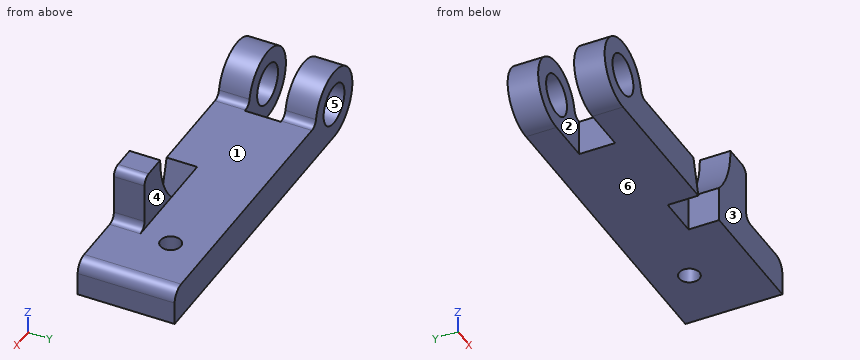
```python
from build123d import *

# Parameters (mm, degrees)
F0_R     = 0.5
F1_DEPTH = 1.1875
F2_W     = 2.274463
F2_H     = 0.879
F2_R     = 0.25
F3_DEPTH = 2.251
F5_DEPTH = 1.625
F7_DEPTH = 0.75
F8_R     = 0.2


with BuildPart() as f1:
    # F0 (on Front) → F1 (new body, symmetric)
    with BuildSketch(Plane.XZ):
        Polygon((-4.03, 0), (-3.03, 0), (-3.03, 0.88), (-4.266, 0.88), align=None)
        with BuildLine():
            Line((-7.646, 0), (-4.03, 0))
            Line((-4.03, 0), (-4.266, 0.88))
            Line((-4.266, 0.88), (-6.58468, 0.88))
            ThreePointArc((-6.58468, 0.88), (-6.712337, 0.92604), (-6.781221, 1.042963))
            ThreePointArc((-6.781221, 1.042963), (-8.323424, 1.441691), (-7.646, 0))
        make_face()
        with Locations((-7.646, 0.88)):
            Circle(F0_R, mode=Mode.SUBTRACT)
        with BuildLine():
            Line((-3.03, 0), (0, 0))
            Line((0, 0), (0, 0.57))
            ThreePointArc((0, 0.57), (-0.090797, 0.789203), (-0.31, 0.88))
            Line((-0.31, 0.88), (-1.737, 0.88))
            Line((-1.737, 0.88), (-1.737, 2.05))
            ThreePointArc((-1.737, 2.05), (-1.795579, 2.191421), (-1.937, 2.25))
            Line((-1.937, 2.25), (-2.487, 2.25))
            ThreePointArc((-2.487, 2.25), (-2.627716, 1.513164), (-3.03, 0.88))
            Line((-3.03, 0.88), (-3.03, 0))
        make_face()
    extrude(amount=F1_DEPTH, both=True)

    # F2 (on Top) → F3 (cut, through all)
    with BuildSketch(Plane.XY):
        with Locations((-7.694299, 0)):
            Rectangle(F2_W, F2_H)
        with Locations((-1.53, 0.3075)):
            Circle(F2_R)
    extrude(amount=F3_DEPTH, mode=Mode.SUBTRACT)

    # F4 (on face) → F5 (cut)
    with BuildSketch(Plane(origin=(0, 1.1875, 0), x_dir=(-1, 0, 0), z_dir=(0, 1, 0))):
        with BuildLine():
            Line((1.737, 0.88), (3.03, 0.88))
            ThreePointArc((3.03, 0.88), (2.627716, 1.513164), (2.487, 2.25))
            Line((2.487, 2.25), (1.937, 2.25))
            ThreePointArc((1.937, 2.25), (1.795579, 2.191421), (1.737, 2.05))
            Line((1.737, 2.05), (1.737, 0.88))
        make_face()
    extrude(amount=-F5_DEPTH, mode=Mode.SUBTRACT)

    # F6 (on face) → F7 (cut)
    with BuildSketch(Plane.XZ.offset(1.1875)):
        Polygon((-3.03, 0), (-3.03, 0.88), (-4.266, 0.88), (-4.03, 0), align=None)
    extrude(amount=-F7_DEPTH, mode=Mode.SUBTRACT)

    # F8
    f8_edges = [f1.edges().sort_by_distance(p)[0] for p in [
        (-1.737, -0.8125, 0.88),
    ]]
    fillet(f8_edges, radius=F8_R)


solid = f1.part
```
Geometry check sheet. Reference: the model listing, model coordinates, mm. Face numbers are marked on the shaded views. A direction names the side the tool comes from. Coordinates: 2 decimals unless noted, no trailing zeros. Order: outer loops, then holes, each group sorted by start corner. A loop starts at its lowest first (then second) coordinate and runs counter-clockwise, first axis right, second up. Notation, with made-up numbers: (12.5, -38) - (19.5, -38) arc R30 ccw to (19.5, -7) - close; hole circle Ø4 at (86, 0.5). An arc over 180 degrees is marked (long way). Answer in a Markdown table with one row per item. Add a question column.
1. Section check D-D (y = 0.2). Enter the section's corners in (x, z).
2. Section check B-B (z = 0.65). Enter the section's corners in (x, y), plus the area to 3 significant figures.
3. Gauge pin test, flat end, axial feed: pin 1 Ø0.6 at (y, z) = (-1, 0) entering from -X. Record the tip position at first contact, or that the pin passes through.
4. Section check A-A (y = -0.95). Enter the section's corners in (x, z), plus the area to 3 significant figures.
5. Draft check along Z on the marked faces 4, 5 and 6. Enter one of: +Z half, -Z half, draft (parallel to the pull), parting line (faces both ways), or undercut.
6. Material ranges on L1, parallel to Y at x = -1.53, z = 0.3; L2, parallel to Z at x = -3.25, y = -0.2; L3, parallel to Y at x = -2.25, z = 1.15, recorded low to high. Write a range as [from, to].
7. Section check C-C (y = 0.9). Enter the section's corners in (x, z).
8. Access from +Z, -Z, +X, -X, +Y, -Y to the whole of each face (thin tool, end or side, straight path). Record for the marked faces 1, 2 and 3.
Data:
| question | item | result |
|---|---|---|
| 1 | outline | (-6.56, 0) - (-1.76, 0) - (-1.76, 0.88) - (-6.56, 0.88) - close; (-1.3, 0) - (0, 0) - (0, 0.57) arc R0.31 ccw to (-0.31, 0.88) - (-1.3, 0.88) - close |
| 2 | outline | (-8.5, -1.19) - (-8.09, -1.19) - (-8.09, -0.44) - (-8.5, -0.44) - close; (-8.5, 0.44) - (-8.09, 0.44) - (-8.09, 1.19) - (-8.5, 1.19) - close; (-7.2, -1.19) - (-4.2, -1.19) - (-4.2, -0.44) - (-3.03, -0.44) - (-3.03, -1.19) - (-0.01, -1.19) - (-0.01, 1.19) - (-7.2, 1.19) - (-7.2, 0.44) - (-6.56, 0.44) - (-6.56, -0.44) - (-7.2, -0.44) - close; hole circle Ø0.5 at (-1.53, 0.31) |
| 2 | area | 16.0 mm² |
| 3 | pin 1 | stops at x = -8.31 |
| 4 | outline | (-7.65, 0) - (-4.03, 0) - (-4.27, 0.88) - (-6.58, 0.88) arc R0.2 cw to (-6.78, 1.04) arc R0.88 ccw (long way) to start; (-3.03, 0) - (0, 0) - (0, 0.57) arc R0.31 ccw to (-0.31, 0.88) - (-1.54, 0.88) arc R0.2 cw to (-1.74, 1.08) - (-1.74, 2.05) arc R0.2 ccw to (-1.94, 2.25) - (-2.49, 2.25) arc R2 cw to (-3.03, 0.88) - close; hole circle Ø1 at (-7.65, 0.88) |
| 4 | area | 8.03 mm² |
| 5 | face 4 | draft |
| 5 | face 5 | undercut |
| 5 | face 6 | -Z half |
| 6 | L1 | y = [-1.19, 0.06], [0.56, 1.19] |
| 6 | L2 | z = [0, 0.88] |
| 6 | L3 | y = [-1.19, -0.44] |
| 7 | outline | (-7.65, 0) - (0, 0) - (0, 0.57) arc R0.31 ccw to (-0.31, 0.88) - (-6.58, 0.88) arc R0.2 cw to (-6.78, 1.04) arc R0.88 ccw (long way) to start; hole circle Ø1 at (-7.65, 0.88) |
| 8 | face 1 | +Z, +Y |
| 8 | face 2 | +Z, -Z, -X |
| 8 | face 3 | +Z, -Z, +X, -X, -Y |
